Source: CAD feature listing. Evaluate the final solid. Frame: model axes, mm. A direction names the side the tool comes from. Give positions to 0.01 mm unless a question says otherwise; leave off trailing zeros. Loops run counter-clockwise (first coordinate to the right, second up) from the corner with the lowest first, then second, coordinate; pieces in that order, holes last. Notation, with made-up numbers: M 68,71 L 116,71 A12 ccw 116,94 Z; hole C 84,-23.75 d5. An arc over 180 degrees is marked long. Answer in a Markdown table with one row per item.
Autodesk Inventor part; units mm, degrees
ref_plane "YZ Plane" through (0, 0, 0) normal (1, 0, 0) x (0, 1, 0)
ref_plane "XZ Plane" through (0, 0, 0) normal (0, 1, 0) x (-1, 0, 0)
ref_plane "XY Plane" through (0, 0, 0) normal (0, 0, 1) x (1, 0, 0)
sketch "Sketch1" plane through (0, 0, 0) normal (0, 1, 0) x (-1, 0, 0)
  line L0 (9.211, 8.9923) -> (-9.839, 8.9923)
  line L1 (-9.839, 8.9923) -> (-9.839, -10.0577)
  line L2 (-9.839, -10.0577) -> (9.211, -10.0577)
  line L3 (9.211, -10.0577) -> (9.211, 8.9923)
  point P0 (0, 0)
  dimension "d0" = 19.05
  dimension "d1" = 19.05
extrude "Extrusion1" add sketch "Sketch1" along normal blind 1.27
sketch "Sketch2" plane through (0, 1.27, 0) normal (0, 1, 0) x (1, 0, 0)
  line L0 (-4.766, -9.0074) -> (5.394, -9.0074)
  line L1 (5.394, -9.0074) -> (5.394, 3.6926)
  line L2 (5.394, 3.6926) -> (-4.766, 3.6926)
  line L3 (-4.766, 3.6926) -> (-4.766, -9.0074)
  line L4 (-9.211, 10.0577) -> (-9.211, -8.9923)
  point P0 (0, 0)
  dimension "d4" = 4.445
  dimension "d5" = 10.16
  dimension "d6" = 12.7
extrude "Extrusion2" cut sketch "Sketch2" against normal up to next
hole "Hole1" at (-2.226, 1.27, -6.2477) direction (0, -1, 0) diameter 1.778 depth 1.27
hole "Hole2" at (2.854, 1.27, -6.2477) direction (0, -1, 0) diameter 1.778 depth 1.27
properties part number "Shutter"
1) Pull-direction query (Z, two-part tool) for faces 1 (the cylindrical face through (-2.83, 0.63, -6.9)), 2 (the flat face through (-7, 1, 8.992)), 3 (the flat face through (-9.211, 1, -1)), 4 (the cylindrical face through (3.395, 0.626, -6.953)); classes: released by +Z, released by -Z, zero draft, split by the parting line, or undercut.
Reply:
| item | result |
|---|---|
| face 1 | undercut |
| face 2 | released by +Z |
| face 3 | zero draft |
| face 4 | undercut |
2) Section A-A, the plane z = -3.25. Return loops of the section in (x, y), then the cut area to 3 significant figures.
Reply:
| item | result |
|---|---|
| outline | M -9.21,0 L -4.77,0 L -4.77,1.27 L -9.21,1.27 Z; M 5.39,0 L 9.84,0 L 9.84,1.27 L 5.39,1.27 Z |
| area | 11.3 mm² |
3) Section B-B, the plane x = 3.5. Return loops of the section in (y, z), then the cut area to 3 significant figures.
Reply:
| item | result |
|---|---|
| outline | M 0,-10.06 L 1.27,-10.06 L 1.27,-6.86 L 0,-6.86 Z; M 0,-5.64 L 1.27,-5.64 L 1.27,-3.69 L 0,-3.69 Z |
| area | 6.53 mm² |
4) Section C-C, the plane y = 1. Return loops of the section in (x, z), then the cut area to 3 significant figures.
Reply:
| item | result |
|---|---|
| outline | M -9.21,-10.06 L 9.84,-10.06 L 9.84,8.99 L 5.39,8.99 L 5.39,-3.69 L -4.77,-3.69 L -4.77,8.99 L -9.21,8.99 Z; hole C -2.23,-6.25 d1.78; hole C 2.85,-6.25 d1.78 |
| area | 229 mm² |
5) Section D-D, the plane x = 0.25. Return loops of the section in (y, z), then the cut area to 3 significant figures.
Reply:
| item | result |
|---|---|
| outline | M 0,-10.06 L 1.27,-10.06 L 1.27,-3.69 L 0,-3.69 Z |
| area | 8.08 mm² |
6) Set-up query: faces 5 (the flat face through (5.394, 1, 3)), 6 (the flat face through (9.839, 1, 0)). Return all of +Z, -Z, +X, -X, +Y, -Y with unobstructed straight access to the full face (end or side cutting, diameter ignored); none if empty.
Reply:
| item | result |
|---|---|
| face 5 | +Z, +Y, -Y |
| face 6 | +Z, -Z, +X, +Y, -Y |
7) Material intervals for L1, parallel to X at y = 0.1, z = 7.75; L2, parallel to X at y = 0.15, z = -7; L3, parallel to Z at x = 0.5, y = 0.6, sorted ascending.
Reply:
| item | result |
|---|---|
| L1 | x = -9.21 to -4.77, 5.39 to 9.84 |
| L2 | x = -9.21 to -2.7, -1.75 to 2.38, 3.33 to 9.84 |
| L3 | z = -10.06 to -3.69 |
